```python
from build123d import *

# Parameters (mm, degrees)
F0_R     = 14.05
F1_DEPTH = 17.1
F2_R     = 2.5
F3_DEPTH = 15
F5_DEPTH = 5


with BuildPart() as f1:
    # F0 (on Top) → F1 (new body)
    with BuildSketch(Plane.XY):
        Circle(F0_R)
    extrude(amount=F1_DEPTH)

    # F2 (on face) → F3 (join)
    with BuildSketch(Plane.XY.offset(17.1)):
        Circle(F2_R)
    extrude(amount=F3_DEPTH)

    # F4 (on face) → F5 (cut)
    with BuildSketch(Plane(origin=(0, 0, 0), x_dir=(1, 0, 0), z_dir=(0, 0, -1))):
        with BuildLine():
            ThreePointArc((-6.275573, 7.159456), (-7.159456, 7.159456), (-7.159456, 6.275573))
            Line((-7.159456, 6.275573), (-6.098796, 5.214913))
            ThreePointArc((-6.098796, 5.214913), (-5.214913, 5.214913), (-5.214913, 6.098796))
            Line((-5.214913, 6.098796), (-6.275573, 7.159456))
        make_face()
        with BuildLine():
            ThreePointArc((7.159456, 6.275573), (7.159456, 7.159456), (6.275573, 7.159456))
            Line((6.275573, 7.159456), (5.214913, 6.098796))
            ThreePointArc((5.214913, 6.098796), (5.214913, 5.214913), (6.098796, 5.214913))
            Line((6.098796, 5.214913), (7.159456, 6.275573))
        make_face()
        with BuildLine():
            ThreePointArc((6.275573, -7.159456), (7.159456, -7.159456), (7.159456, -6.275573))
            Line((7.159456, -6.275573), (6.098796, -5.214913))
            ThreePointArc((6.098796, -5.214913), (5.214913, -5.214913), (5.214913, -6.098796))
            Line((5.214913, -6.098796), (6.275573, -7.159456))
        make_face()
        with BuildLine():
            ThreePointArc((-7.159456, -6.275573), (-7.159456, -7.159456), (-6.275573, -7.159456))
            Line((-6.275573, -7.159456), (-5.214913, -6.098796))
            ThreePointArc((-5.214913, -6.098796), (-5.214913, -5.214913), (-6.098796, -5.214913))
            Line((-6.098796, -5.214913), (-7.159456, -6.275573))
        make_face()
    extrude(amount=-F5_DEPTH, mode=Mode.SUBTRACT)


solid = f1.part
```
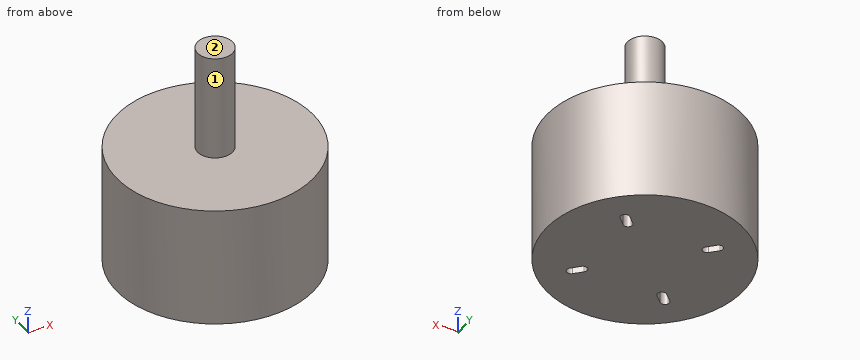
Model file for the job. Use its own axes, mm. Face numbers are marked on the shaded views. A direction names the side the tool comes from. Give positions to 0.01 mm unless a question says otherwise; leave off trailing zeros. Loops run counter-clockwise (first coordinate to the right, second up) from the corner with the lowest first, then second, coordinate; pieces in that order, holes last. Notation, with made-up numbers: (47.25, -27) - (84.25, -27) arc R20 cw to (84.25, -5) - close; hole circle Ø8 at (42, -17.5). An arc over 180 degrees is marked (long way). One line per item, written item: value. Start each with the question number.
1. Which spindle directions (+Z, -Z, +X, -X, +Y, -Y) get a long thin tool onto all of the face, cutting with end or side? Do the marked faces 1 and 2. Say none if no direction does.
2. Slice it at D-D (z = 22.5). List the corners of the cut face in (x, y).
3. Slice it at C-C (z = 10). List the corners of the cut face in (x, y), plus the area to 3 significant figures.
4. Probe L1, parallel to Z at x = 7.5, y = -1; L2, parallel to X at y = -1, z = 3; L3, parallel to X at y = 10.5, z = 6. List the from-to ranges inside material, lowest first. Write a range as from..to.
5. Pin check, flat tips, straight feed: pin 1 (5 mm diameter, centred on x = 6, y = 4.5, fed in from -Z); pin 2 (1.5 mm diameter, centred on y = 4.5, z = 18, fed in from +X) (3 decimals); pin 3 (8 mm diameter, centred on x = -9.5, z = 13.5, fed in from +Y); pin 4 (6 mm diameter, centred on x = 5, z = 21.5, fed in from +Y). Stop position of each tip, or through.
6. Slice it at A-A (y = 0). List the corners of the cut face in (x, z), plus the area to 3 significant figures.
Solution:
1. face 1: +Z
1. face 2: +Z, +X, -X, +Y, -Y
2. outline: circle Ø5 at (0, 0)
3. outline: circle Ø28.1 at (0, 0)
3. area: 620 mm^2
4. L1: z = 0..17.1
4. L2: x = -14.01..14.01
4. L3: x = -9.34..9.34
5. pin 1: stops at z = 0
5. pin 2: passes through
5. pin 3: stops at y = 12.93
5. pin 4: stops at y = 1.5
6. outline: (-14.05, 0) - (14.05, 0) - (14.05, 17.1) - (2.5, 17.1) - (2.5, 32.1) - (-2.5, 32.1) - (-2.5, 17.1) - (-14.05, 17.1) - close
6. area: 556 mm^2
